```python
from build123d import *

# Parameters (mm, degrees)
SKETCH1_R           = 1
BOSS_EXTRUDE1_DEPTH = 3
SKETCH3_W           = 1
SKETCH3_H           = 2
MIRROR1_OUTLINE_R   = 1
MIRROR1_DEPTH       = 3
MIRROR1_START       = 2
MIRROR1_2_DEPTH     = 1


# Read off the part's stored shape, not the designer's step: Mirror1
with BuildPart() as part:
    # Sketch1 → Boss-Extrude1 (new body)
    with BuildSketch(Plane(origin=(0, 0, 0), x_dir=(1, 0, 0), z_dir=(0, 1, 0))):
        with BuildLine():
            Line((0, 0), (22, 0))
            Line((22, 0), (22, 8))
            ThreePointArc((22, 8), (12.100505063, 12.100505063), (8, 22))
            Line((8, 22), (0, 22))
            Line((0, 22), (0, 0))
        make_face()
        with Locations(Location((3, 3, 0), (0, 0, 270))):
            Circle(SKETCH1_R, mode=Mode.SUBTRACT)
    extrude(amount=BOSS_EXTRUDE1_DEPTH)

    # Sketch3 → Cut-Revolve1 (revolve, cut)
    with BuildSketch(Plane(origin=(22, 0, 0), x_dir=(0, 0, -1), z_dir=(1, 0, 0))):
        with Locations((7.5, 1)):
            Rectangle(SKETCH3_W, SKETCH3_H)
    revolve(axis=Axis((22, 7.36812707, -22), (0, -1, 0)), mode=Mode.SUBTRACT)

    # Mirror1 outline → Mirror1 (add)
    with BuildSketch(Plane(origin=(0, 0, 0), x_dir=(1, 0, 0), z_dir=(0, 1, 0))):
        with BuildLine():
            Line((0, 44), (0, 22))
            Line((0, 22), (7, 22))
            ThreePointArc((7, 22), (32.606601718, 32.606601718), (22, 7))
            Line((22, 7), (22, 0))
            Line((22, 0), (44, 0))
            Line((44, 0), (44, 44))
            Line((44, 44), (0, 44))
        make_face()
        with Locations((41, 3)):
            Circle(MIRROR1_OUTLINE_R, mode=Mode.SUBTRACT)
        with Locations((3, 41)):
            Circle(MIRROR1_OUTLINE_R, mode=Mode.SUBTRACT)
        with Locations((41, 41)):
            Circle(MIRROR1_OUTLINE_R, mode=Mode.SUBTRACT)
    extrude(amount=MIRROR1_DEPTH)

    # Mirror1 2 outline → Mirror1 2 (add)
    with BuildSketch(Plane(origin=(0, 0, 0), x_dir=(1, 0, 0), z_dir=(0, 1, 0)).offset(MIRROR1_START)):
        with BuildLine():
            ThreePointArc((22, 7), (32.606601718, 32.606601718), (7, 22))
            Line((7, 22), (8, 22))
            ThreePointArc((8, 22), (31.899494937, 31.899494937), (22, 8))
            Line((22, 8), (22, 7))
        make_face()
    extrude(amount=MIRROR1_2_DEPTH)


solid = part.part
```
Geometry: final body of the model. Coordinates: model frame, mm. Coordinates: 2 decimals unless noted, no trailing zeros. Order: outer loops, then holes, each group sorted by start corner. A loop starts at its lowest first (then second) coordinate and runs counter-clockwise, first axis right, second up. Notation, with made-up numbers: (69.5, 31) - (75.5, 31) arc R21 cw to (75.5, 46) - close; hole circle Ø9 at (85.5, 4.5). An arc over 180 degrees is marked (long way). Return JSON: item names as keys, results as strings. Group by question number.
1. Cut plane B-B (y = 2.5). Output: boundary loops of the cut face in (x, z).
2. Cut plane D-D (z = -29). Output: boundary loops of the cut face in (x, y).
3. Cut plane A-A (z = -41). Output: boundary loops of the cut face in (x, y).
4. Pull-direction query (X, two-part tool) for faces 1 (the face through (3.676, 1.479, -3.737)), 2 (the face through (44, 1, -22)), 3 (the face through (22, 1, -44)); classes: pulls with the +X half, pulls with the -X half, needs draft (parallel to the pull), parting line crosses it, or undercut.
5. Cut plane C-C (x = 41). Output: boundary loops of the cut face in (y, z).
6. Material intervals for line 1 along X through (y, z) = (2.2, -3); line 2 along Z through (x, y) = (41, 1.4); line 3 along Z through (x, y) = (22, 1.2), sorted ascending. Write a range as [from, to].
7. Pin query (flat end, axial travel): pin 1 (9 mm diameter, centred on x = 22.5, z = -27, fed in from -Y). Return the tip coordinate at first contact, or that it passes through.
Resolved:
{
 "1": {"outline": "(0, -44) - (44, -44) - (44, 0) - (0, 0) - close; hole circle Ø2 at (3, -41); hole circle Ø2 at (3, -3); hole circle Ø28 at (22, -22); hole circle Ø2 at (41, -41); hole circle Ø2 at (41, -3)"},
 "2": {"outline": "(0, 0) - (8.73, 0) - (8.73, 2) - (9.88, 2) - (9.88, 3) - (0, 3) - close; (34.12, 2) - (35.27, 2) - (35.27, 0) - (44, 0) - (44, 3) - (34.12, 3) - close"},
 "3": {"outline": "(0, 0) - (2, 0) - (2, 3) - (0, 3) - close; (4, 0) - (40, 0) - (40, 3) - (4, 3) - close; (42, 0) - (44, 0) - (44, 3) - (42, 3) - close"},
 "4": {"face 1": "undercut", "face 2": "pulls with the +X half", "face 3": "needs draft"},
 "5": {"outline": "(0, -44) - (3, -44) - (3, -42) - (0, -42) - close; (0, -40) - (3, -40) - (3, -4) - (0, -4) - close; (0, -2) - (3, -2) - (3, 0) - (0, 0) - close"},
 "6": {"line 1": "x = [0, 2], [4, 40], [42, 44]", "line 2": "z = [-44, -42], [-40, -4], [-2, 0]", "line 3": "z = [-44, -37], [-7, 0]"},
 "7": {"pin 1": "passes through"}
}
